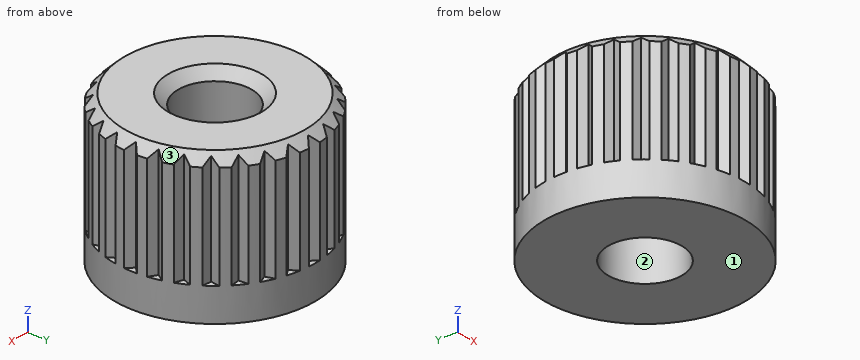
from build123d import *

# Parameters (mm, degrees)
SKETCH026_R                 = 3
PAD002001003004001006_DEPTH = 4.4
SKETCH027_R                 = 1.1
POCKET011_DEPTH             = 4.401
CHAMFER_SIZE                = 0.3
POCKET012_DEPTH             = 3.4
POLARPATTERN_COUNT          = 28
CHAMFER001_SIZE             = 0.3


with BuildPart() as part:
    # Sketch026 → Pad002001003004001006 (new body)
    with BuildSketch(Plane.XY):
        Circle(SKETCH026_R)
    extrude(amount=PAD002001003004001006_DEPTH)

    # Sketch027 (on Face3 of Pad002001003004001006) → Pocket011 (cut, through all)
    with BuildSketch(Plane.XY.offset(4.4)):
        Circle(SKETCH027_R)
    extrude(amount=-POCKET011_DEPTH, mode=Mode.SUBTRACT)

    # Chamfer
    chamfer_edges = [part.edges().sort_by_distance(p)[0] for p in [
        (-3, 0, 4.4),
    ]]
    chamfer(chamfer_edges, length=CHAMFER_SIZE)

    # Sketch028 (on Face4 of Chamfer) → Pocket012 (cut)
    with BuildSketch(Plane.XY.offset(4.4)):
        Polygon((-0.2, 3), (0, 2.8), (0.2, 3), align=None)
    pocket012 = extrude(amount=-POCKET012_DEPTH, mode=Mode.SUBTRACT)

    # PolarPattern: Pocket012 ×28 about axis
    polarpattern_axis = Axis((0, 0, 4.4), (0, 0, 1))
    for i in range(1, POLARPATTERN_COUNT):
        add(pocket012.rotate(polarpattern_axis, i * 360 / POLARPATTERN_COUNT), mode=Mode.SUBTRACT)

    # Chamfer001
    chamfer001_edges = [part.edges().sort_by_distance(p)[0] for p in [
        (-1.1, 0, 4.4),
    ]]
    chamfer(chamfer001_edges, length=CHAMFER001_SIZE)


solid = part.part
Model file for the job. Use its own axes, mm. Face numbers are marked on the shaded views. Round coordinates to 2 decimals unless told otherwise and drop trailing zeros. Write each question's results on one line, items separated by ' | '.
(1) Pin check, flat tip, straight feed: pin 1 (1.5 mm diameter, centred on x = -1, z = 1.5, fed in from -Y). Stop position of the tip, or through.
Answer below:
pin 1: stops at y = -2.99
(2) Mould opens along Y. For the marked faces 1, 2 and 3 say: released by +Y, released by -Y, zero draft, split by the parting line, or undercut.
Answer below:
face 1: zero draft | face 2: undercut | face 3: split by the parting line
(3) Wall check: L1, parallel to Y at x = -0.05, z = 1.7; L2, parallel to X at y = -0.8, z = 2.45; L3, parallel to X at y = 0.1, z = 2.15. Give the ranges that are in metal, low to high.
Answer below:
L1: y = -2.85 to -1.1, 1.1 to 2.85 | L2: x = -2.84 to -0.75, 0.75 to 2.84 | L3: x = -2.9 to -1.1, 1.1 to 2.9
